Study the drawing (mm; zero at the part's minimum x, y, z) and answer. Coordinates: 2 decimals unless noted, no trailing zeros. Order: outer loops, then holes, each group sorted by start corner. A loop starts at its lowest first (then second) coordinate and runs counter-clockwise, first axis right, second up. Notation, with made-up numbers: (38.5, 8.25) - (66.5, 8.25) arc R21 cw to (66.5, 43.25) - close; hole circle Ø1 at (7.5, 46). An arc over 180 degrees is marked (long way). Write item = value, one per line.
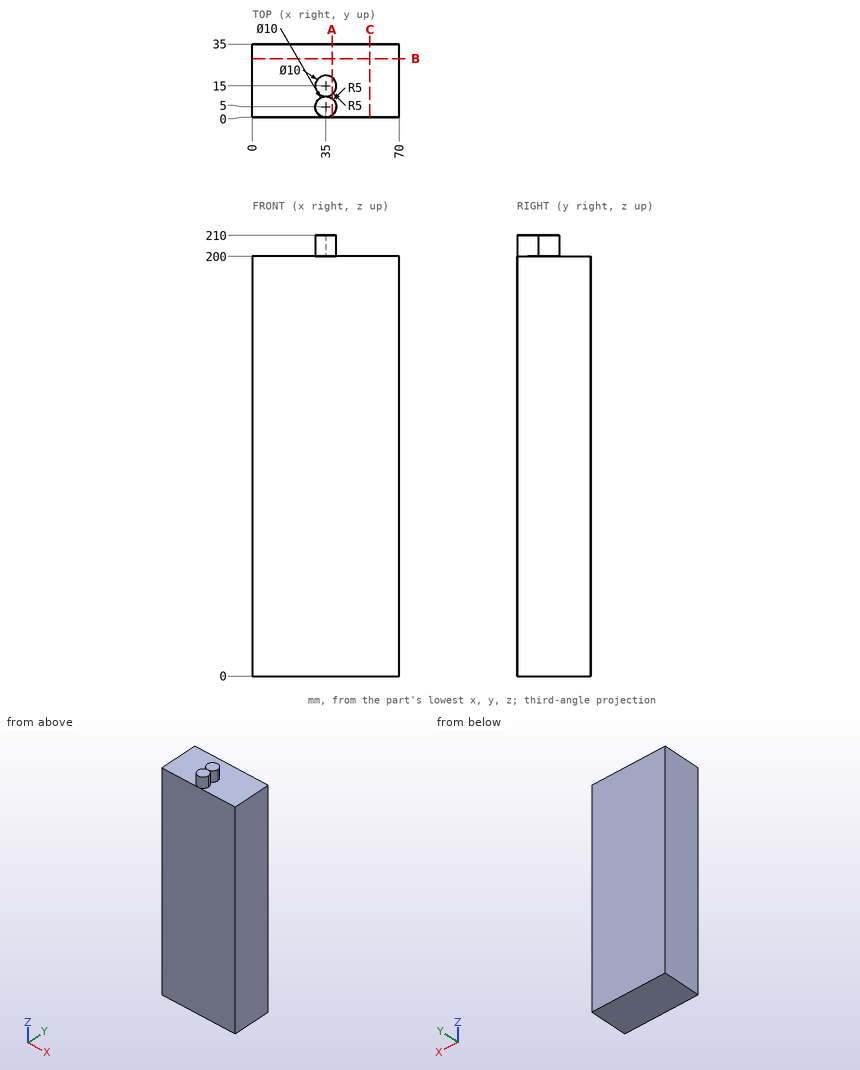
1) The part is cut by section A-A (x = 38). Determine the outline of the cut face in (y, z).
Returned:
outline = (0, 0) - (35, 0) - (35, 200) - (19, 200) - (19, 210) - (11, 210) - (11, 200) - (9, 200) - (9, 210) - (1, 210) - (1, 200) - (0, 200) - close
2) The part is cut by section B-B (y = 28). Determine the outline of the cut face in (x, z).
Returned:
outline = (0, 0) - (70, 0) - (70, 200) - (0, 200) - close
3) A straight line is drawn through the part: line 1 along Z through (x, y) = (4.5, 22). Find the intervals that lie inside material, in ascending order. Write a range as from..to.
Returned:
line_1 = 0..200
4) The part is cut by section C-C (x = 56). Determine the outline of the cut face in (y, z), and give its area (3 significant figures).
Returned:
outline = (0, 0) - (35, 0) - (35, 200) - (0, 200) - close
area = 7,000 mm^2
5) A flat-ended cylindrical pin translates along its axis: pin 1 Ø17.5 at (x, y) = (20.5, 14.5) entering from +Z. Find the tip coordinate at first contact, or state that the pin passes through.
Returned:
pin_1 = 200
